```python
from build123d import *

# Parameters (mm, degrees)
BOSS_EXTRUDE1_DEPTH           = 3
BOSS_EXTRUDE2_DEPTH           = 18
CUT_EXTRUDE1_DEPTH            = 18
FILLET2_R                     = 0.5
BOSS_EXTRUDE3_DEPTH           = 4
BOSS_EXTRUDE4_START           = 3
BOSS_EXTRUDE4_DEPTH           = 5
SKETCH6_W                     = 2
SKETCH6_H                     = 4
SKETCH6_W_2                   = 1.5
SKETCH6_H_2                   = 3.5
BOSS_EXTRUDE5_DEPTH           = 14
SKETCH7_W                     = 1.5
SKETCH7_H                     = 3.5
BOSS_EXTRUDE6_DEPTH           = 2
BOSS_EXTRUDE6_DRAFT           = 16
SKETCH7_W_2                   = 2
SKETCH7_H_2                   = 4
BOSS_EXTRUDE6_PROFILE_2_DEPTH = 2
BOSS_EXTRUDE6_PROFILE_2_DRAFT = 16
BOSS_EXTRUDE6_PROFILE_3_DEPTH = 2
BOSS_EXTRUDE6_PROFILE_3_DRAFT = 16
SKETCH8_W                     = 1.5
SKETCH8_H                     = 6.35
BOSS_EXTRUDE7_DEPTH           = 7.5
FILLET3_R                     = 1
SKETCH9_R                     = 1.75
CUT_EXTRUDE2_DEPTH            = 11


with BuildPart() as part:
    # Sketch1 → Boss-Extrude1 (new body)
    with BuildSketch(Plane.XY):
        with BuildLine():
            Line((-13, -11.5), (13, -11.5))
            ThreePointArc((13, -11.5), (14.414213562, -10.914213562), (15, -9.5))
            Line((15, -9.5), (15, 9.5))
            ThreePointArc((15, 9.5), (14.414213562, 10.914213562), (13, 11.5))
            Line((13, 11.5), (-13, 11.5))
            ThreePointArc((-13, 11.5), (-14.414213562, 10.914213562), (-15, 9.5))
            Line((-15, 9.5), (-15, -9.5))
            ThreePointArc((-15, -9.5), (-14.414213562, -10.914213562), (-13, -11.5))
        make_face()
    extrude(amount=BOSS_EXTRUDE1_DEPTH)

    # Sketch2 → Boss-Extrude2 (add)
    with BuildSketch(Plane(origin=(0, 0, 0), x_dir=(-1, 0, 0), z_dir=(0, 0, -1))):
        with BuildLine():
            Line((-7.244277484, 9.271690642), (-12.709444213, 4.557717215))
            ThreePointArc((-12.709444213, 4.557717215), (-13.477483514, 3.535359867), (-13.75, 2.286026573))
            Line((-13.75, 2.286026573), (-13.75, -7))
            ThreePointArc((-13.75, -7), (-12.871320344, -9.121320344), (-10.75, -10))
            Line((-10.75, -10), (10.75, -10))
            ThreePointArc((10.75, -10), (12.871320344, -9.121320344), (13.75, -7))
            Line((13.75, -7), (13.75, 2.286026573))
            ThreePointArc((13.75, 2.286026573), (13.477483514, 3.535359867), (12.709444213, 4.557717215))
            Line((12.709444213, 4.557717215), (7.244277484, 9.271690642))
            ThreePointArc((7.244277484, 9.271690642), (6.330043315, 9.812034133), (5.28483327, 10))
            Line((5.28483327, 10), (-5.28483327, 10))
            ThreePointArc((-5.28483327, 10), (-6.330043315, 9.812034133), (-7.244277484, 9.271690642))
        make_face()
    extrude(amount=BOSS_EXTRUDE2_DEPTH)

    # Sketch3 → Cut-Extrude1 (cut)
    with BuildSketch(Plane.XY.offset(3)):
        with BuildLine():
            Line((11.403148071, 3.043256787), (5.937981342, 7.757230214))
            ThreePointArc((5.937981342, 7.757230214), (5.633236618, 7.937344711), (5.28483327, 8))
            Line((5.28483327, 8), (-5.28483327, 8))
            ThreePointArc((-5.28483327, 8), (-5.633236618, 7.937344711), (-5.937981342, 7.757230214))
            Line((-5.937981342, 7.757230214), (-11.403148071, 3.043256787))
            ThreePointArc((-11.403148071, 3.043256787), (-11.659161171, 2.702471004), (-11.75, 2.286026573))
            Line((-11.75, 2.286026573), (-11.75, -7))
            ThreePointArc((-11.75, -7), (-11.457106781, -7.707106781), (-10.75, -8))
            Line((-10.75, -8), (10.75, -8))
            ThreePointArc((10.75, -8), (11.457106781, -7.707106781), (11.75, -7))
            Line((11.75, -7), (11.75, 2.286026573))
            ThreePointArc((11.75, 2.286026573), (11.659161171, 2.702471004), (11.403148071, 3.043256787))
        make_face()
    extrude(amount=-CUT_EXTRUDE1_DEPTH, mode=Mode.SUBTRACT)

    # Fillet2
    fillet2_edges = [part.edges().sort_by_distance(p)[0] for p in [
        (14.414213562, -10.914213562, 3),
        (15, 0, 3),
        (14.414213562, 10.914213562, 3),
        (0, 11.5, 3),
        (-14.414213562, 10.914213562, 3),
        (-15, 0, 3),
        (9.976860849, 6.914703929, -18),
        (13.75, -2.356986713, -18),
        (12.871320344, -9.121320344, -18),
        (-13.477483514, 3.535359867, -18),
        (-9.976860849, 6.914703929, -18),
        (-6.330043315, 9.812034133, -18),
        (0, 10, -18),
        (6.330043315, 9.812034133, -18),
        (13.477483514, 3.535359867, -18),
        (0, -10, -18),
        (-12.871320344, -9.121320344, -18),
        (-13.75, -2.356986713, -18),
        (-14.414213562, -10.914213562, 3),
        (11.659161171, 2.702471004, 3),
        (8.670564706, 5.400243501, 3),
        (5.633236618, 7.937344711, 3),
        (0, 8, 3),
        (-5.633236618, 7.937344711, 3),
        (-8.670564706, 5.400243501, 3),
        (-11.659161171, 2.702471004, 3),
        (-11.75, -2.356986713, 3),
        (-11.457106781, -7.707106781, 3),
        (0, -8, 3),
        (11.457106781, -7.707106781, 3),
        (11.75, -2.356986713, 3),
        (0, -11.5, 3),
    ]]
    fillet(fillet2_edges, radius=FILLET2_R)

    # Sketch4 → Boss-Extrude3 (add, symmetric)
    with BuildSketch(Plane(origin=(0, 0, 0), x_dir=(0, 0, -1), z_dir=(1, 0, 0))):
        Polygon((2.5, 10), (2.5, 11.5), (12.788235775, 10), align=None)
    extrude(amount=BOSS_EXTRUDE3_DEPTH, both=True)

    # Sketch5 → Boss-Extrude4 (add)
    with BuildSketch(Plane(origin=(0, 0, 0), x_dir=(0, 0, -1), z_dir=(1, 0, 0)).offset(BOSS_EXTRUDE4_START)):
        Polygon((2.5, -10), (12.788235775, -10), (2.5, -11.5), align=None)
    boss_extrude4 = extrude(amount=BOSS_EXTRUDE4_DEPTH)

    # Mirror1: Boss-Extrude4 across plane
    add(boss_extrude4.mirror(Plane(origin=(0, 0, 0), x_dir=(0, 0, 1), z_dir=(1, 0, 0))))

    # Sketch6 → Boss-Extrude5 (add)
    with BuildSketch(Plane.XY.offset(-15)):
        with Locations((0, 3.188606821)):
            Rectangle(SKETCH6_W, SKETCH6_H)
        with Locations((-5.961546064, -3.204394816)):
            Rectangle(SKETCH6_W_2, SKETCH6_H_2)
        with Locations((5.961546064, -3.204394816)):
            Rectangle(SKETCH6_W_2, SKETCH6_H_2)
    extrude(amount=BOSS_EXTRUDE5_DEPTH)


with BuildPart() as boss_extrude6_tool:
    # Sketch7 → Boss-Extrude6 (with draft: the straight prism first)
    with BuildSketch(Plane.XY.offset(-1)):
        with Locations((-5.961546064, -3.204394816)):
            Rectangle(SKETCH7_W, SKETCH7_H)
    extrude(amount=BOSS_EXTRUDE6_DEPTH)
    # Boss-Extrude6: the draft: its side faces are tilted about the plane it starts from
    boss_extrude6_sides = [boss_extrude6_tool.faces().sort_by_distance(p)[0] for p in [
        (-5.211546064, -3.204394816, 0),
        (-5.961546064, -1.454394816, 0),
        (-6.711546064, -3.204394816, 0),
        (-5.961546064, -4.954394816, 0),
    ]]
    draft(boss_extrude6_sides, Plane.XY.offset(-1), BOSS_EXTRUDE6_DRAFT)


with BuildPart() as part_1:
    add(part.part)

    # Boss-Extrude6: add boss_extrude6_tool
    add(boss_extrude6_tool.part)


with BuildPart() as boss_extrude6_profile_2_tool:
    # Sketch7 → Boss-Extrude6 profile 2 (with draft: the straight prism first)
    with BuildSketch(Plane.XY.offset(-1)):
        with Locations((0, 3.188606821)):
            Rectangle(SKETCH7_W_2, SKETCH7_H_2)
    extrude(amount=BOSS_EXTRUDE6_PROFILE_2_DEPTH)
    # Boss-Extrude6 profile 2: the draft: its side faces are tilted about the plane it starts from
    boss_extrude6_profile_2_sides = [boss_extrude6_profile_2_tool.faces().sort_by_distance(p)[0] for p in [
        (-1, 3.188606821, 0),
        (0, 1.188606821, 0),
        (1, 3.188606821, 0),
        (0, 5.188606821, 0),
    ]]
    draft(boss_extrude6_profile_2_sides, Plane.XY.offset(-1), BOSS_EXTRUDE6_PROFILE_2_DRAFT)


with BuildPart() as part_2:
    add(part_1.part)

    # Boss-Extrude6 profile 2: add boss_extrude6_profile_2_tool
    add(boss_extrude6_profile_2_tool.part)


with BuildPart() as boss_extrude6_profile_3_tool:
    # Sketch7 → Boss-Extrude6 profile 3 (with draft: the straight prism first)
    with BuildSketch(Plane.XY.offset(-1)):
        with Locations((5.961546064, -3.204394816)):
            Rectangle(SKETCH7_W, SKETCH7_H)
    extrude(amount=BOSS_EXTRUDE6_PROFILE_3_DEPTH)
    # Boss-Extrude6 profile 3: the draft: its side faces are tilted about the plane it starts from
    boss_extrude6_profile_3_sides = [boss_extrude6_profile_3_tool.faces().sort_by_distance(p)[0] for p in [
        (6.711546064, -3.204394816, 0),
        (5.961546064, -1.454394816, 0),
        (5.211546064, -3.204394816, 0),
        (5.961546064, -4.954394816, 0),
    ]]
    draft(boss_extrude6_profile_3_sides, Plane.XY.offset(-1), BOSS_EXTRUDE6_PROFILE_3_DRAFT)


with BuildPart() as part_3:
    add(part_2.part)

    # Boss-Extrude6 profile 3: add boss_extrude6_profile_3_tool
    add(boss_extrude6_profile_3_tool.part)

    # Sketch8 → Boss-Extrude7 (add)
    with BuildSketch(Plane(origin=(0, 0, -18), x_dir=(-1, 0, 0), z_dir=(0, 0, -1))):
        with Locations((0, 3.188606821)):
            Rectangle(SKETCH8_W, SKETCH8_H)
        with Locations((-5.961546064, -3.204394816)):
            Rectangle(SKETCH8_W, SKETCH8_H)
        with Locations((5.961546064, -3.204394816)):
            Rectangle(SKETCH8_W, SKETCH8_H)
    extrude(amount=BOSS_EXTRUDE7_DEPTH)

    # Fillet3
    fillet3_edges = [part_3.edges().sort_by_distance(p)[0] for p in [
        (0, 0.013606821, -25.5),
        (0, 6.363606821, -25.5),
        (5.961546064, -6.379394816, -25.5),
        (5.961546064, -0.029394816, -25.5),
        (-5.961546064, -6.379394816, -25.5),
        (-5.961546064, -0.029394816, -25.5),
    ]]
    fillet(fillet3_edges, radius=FILLET3_R)

    # Sketch9 → Cut-Extrude2 (cut, symmetric)
    with BuildSketch(Plane(origin=(0.75, 0, 0), x_dir=(0, 0, -1), z_dir=(1, 0, 0))):
        with Locations(Location((22.325, 3.188606821, 0), (0, 0, 90))):
            Circle(SKETCH9_R)
        with Locations(Location((22.325, -3.204394816, 0), (0, 0, 90))):
            Circle(SKETCH9_R)
    extrude(amount=CUT_EXTRUDE2_DEPTH, both=True, mode=Mode.SUBTRACT)


solid = part_3.part
```
The listing builds one solid part. Answer for the finished solid, in the listing's coordinates (mm). A direction names the side the tool comes from. Round coordinates to 2 decimals unless told otherwise and drop trailing zeros. Loops run counter-clockwise (first coordinate to the right, second up) from the corner with the lowest first, then second, coordinate; pieces in that order, holes last.
Q1. Find the intervals of material crossed by line 1 (X direction, y = -4.75, z = -13); line 2 (X direction, y = 1.25, z = 0.75); line 3 (X direction, y = -6, z = -7.25), in increasing order.
Q2. Section B-B, the plane z = -21 is taken. Determine the outline of the cut face in (x, y).
Q3. For a pull along X with two mould halves and no side action, classify faces 1 (the face through (13.47, 3.55, -8.63)), 2 (the face through (-10.02, 6.88, -8.63)), 3 (the face through (-6, -3, -25.5)), 4 (the face through (5.212, -3, -20)) as released by +X, released by -X, zero draft, split by the parting line, or undercut.
Q4. Section D-D, the plane y = 0.5 is taken. Determine the outline of the cut face in (x, z).
Q5. Which of the six approach directions +Z, -Z, +X, -X, +Y, -Y give full straight-line access (tool end or side, diameter ignored) to faces 5 (the face through (-0.75, 3, -20)), 6 (the face through (-6.34, 9.81, -8.63)), 7 (the face through (-5.212, -3, -20)), 8 (the face through (-6, -1.454, -8))?
Q6. Given pin 1 Ø5 at (x, z) = (0.5, -8) entering from +Y; pin 2 Ø6 at (x, z) = (3.5, -10.5) entering from -Y; pin 3 Ø2 at (y, z) = (3, -4.5) entering from -X, each flat-ended and moving along its own axis, determine where each tip first touches the part or whether it passes through.
Q7. Section A-A, the plane z = -1.5 is taken. Count the separate pieces of the cut face and the enclosed holes in it, then the cut area to 3 significant figures.
Completed:
1. line 1: x = -13.75 to -11.75, -6.71 to -5.21, 5.21 to 6.71, 11.75 to 13.75
1. line 2: x = -15 to -11.75, 11.75 to 15
1. line 3: x = -13.75 to -11.75, 11.75 to 13.75
2. outline: (-6.71, -6.38) - (-5.21, -6.38) - (-5.21, -4.35) - (-6.71, -4.35) - close; (-6.71, -2.06) - (-5.21, -2.06) - (-5.21, -0.03) - (-6.71, -0.03) - close; (-0.75, 0.01) - (0.75, 0.01) - (0.75, 2.05) - (-0.75, 2.05) - close; (-0.75, 4.33) - (0.75, 4.33) - (0.75, 6.36) - (-0.75, 6.36) - close; (5.21, -6.38) - (6.71, -6.38) - (6.71, -4.35) - (5.21, -4.35) - close; (5.21, -2.06) - (6.71, -2.06) - (6.71, -0.03) - (5.21, -0.03) - close
3. face 1: released by +X
3. face 2: released by -X
3. face 3: zero draft
3. face 4: undercut
4. outline: (-15, 0) - (-13.75, 0) - (-13.75, -17.5) arc R0.5 ccw to (-13.25, -18) - (-0.75, -18) - (-0.75, -25.36) - (0.75, -25.36) - (0.75, -18) - (13.25, -18) arc R0.5 ccw to (13.75, -17.5) - (13.75, 0) - (15, 0) - (15, 2.5) arc R0.5 ccw to (14.5, 3) - (12.25, 3) arc R0.5 ccw to (11.75, 2.5) - (11.75, -15) - (-11.75, -15) - (-11.75, 2.5) arc R0.5 ccw to (-12.25, 3) - (-14.5, 3) arc R0.5 ccw to (-15, 2.5) - close
5. face 5: -Z, -X, +Y, -Y
5. face 6: -Z, -X, +Y
5. face 7: -Z, +Y, -Y
5. face 8: +Z
6. pin 1: stops at y = 11.06
6. pin 2: stops at y = -10.77
6. pin 3: stops at x = -13.75
7. separate pieces: 4
7. enclosed holes: 1
7. area: 174 mm2
